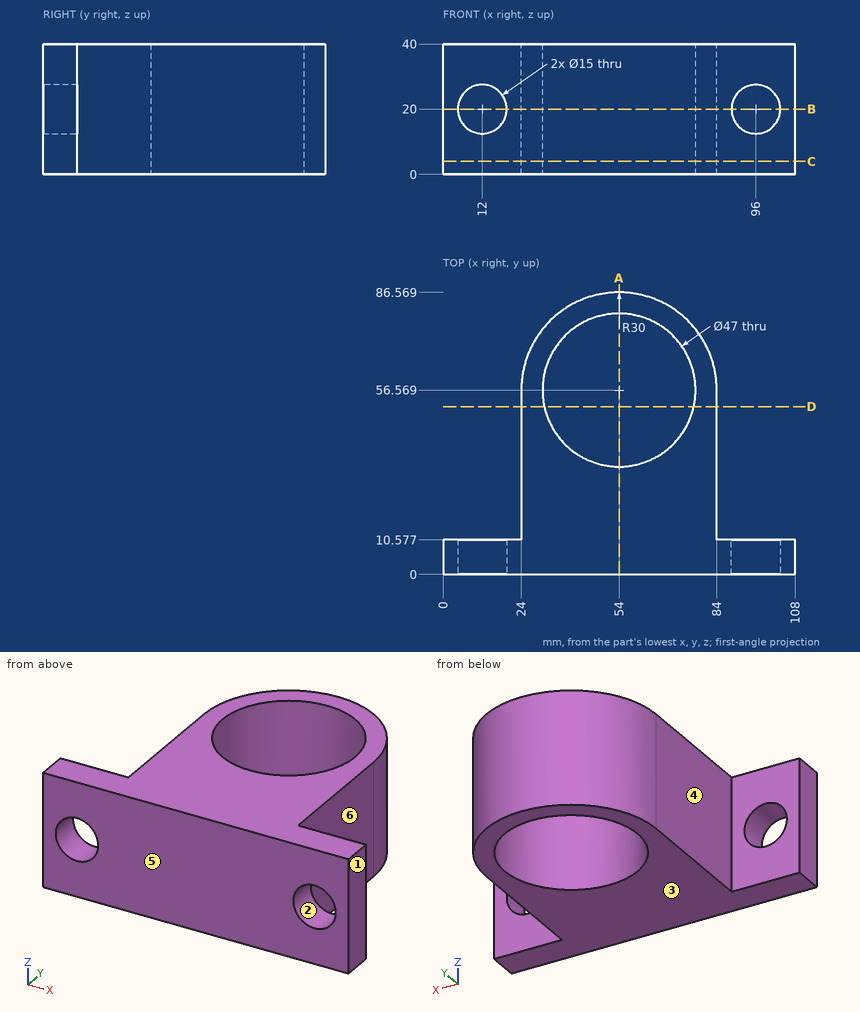
Job drawing, mm, ordinate dimensions from the low corner. One solid piece. A direction names the side the tool comes from. Coordinates: 2 decimals unless noted, no trailing zeros. Write each loop counter-clockwise with the first axis right and the second up, starting at its lowest first coordinate (ties: lowest second). Pieces come first, ordered by that corner, then holes. Notation, with made-up numbers: (-30.5, -12) - (7.5, -12) arc R33 cw to (7.5, 19) - close; hole circle Ø1 at (63.25, 89). An arc over 180 degrees is marked (long way). Use a Markdown table: item, result. Add a question column.
Item 1: Band-saw the part on B-B, the plane z = 20. Give the cut face in (x, y), and give its area (3 significant figures).
Item 2: 3-axis set-ups, long thin cutter, end or side, ignore diameter. For the marked faces 4, 5 and 6: which of +Z, -Z, +X, -X, +Y, -Y reach the whole face in a straight line?
Item 3: Band-saw the part on C-C, the plane z = 4. Give the cut face in (x, y).
Item 4: Flat gauge pins, fed straight in: pin 1 (1.5 mm diameter, centred on y = 66.5, z = 7, fed in from +X); pin 2 (10 mm diameter, centred on x = 39.5, y = 75, fed in from -Z); pin 3 (19 mm diameter, centred on x = 17.5, z = 26.5, fed in from +Y) (1 decimal); pin 4 (8 mm diameter, centred on y = 23.5, z = 7.5, fed in from -X). Where does each tip first touch, or does it go through?
Item 5: Band-saw the part on A-A, the plane x = 54. Give the cut face in (y, z).
Item 6: Mould opens along Z. For the marked faces 1, 2 and 3 say: pulls with the +Z half, pulls with the -Z half, needs draft (parallel to the pull), parting line crosses it, or undercut.
Item 7: Band-saw the part on D-D, the plane y = 51.5. Give the cut face in (x, z).
Item 8: Drill centre lines: L1, parallel to X at y = 8.75, z = 20; L2, parallel to Z at x = 96, y = 3; L3, parallel to X at y = 23, z = 7. Where is each one in solid material? Low to high. Write a range as from..to.
Numbers:
| question | item | result |
|---|---|---|
| 1 | outline | (0, 0) - (4.5, 0) - (4.5, 10.58) - (0, 10.58) - close; (19.5, 0) - (88.5, 0) - (88.5, 10.58) - (84, 10.58) - (84, 56.57) arc R30 ccw to (24, 56.57) - (24, 10.58) - (19.5, 10.58) - close; (103.5, 0) - (108, 0) - (108, 10.58) - (103.5, 10.58) - close; hole circle Ø47 at (54, 56.57) |
| 1 | area | 3,260 mm2 |
| 2 | face 4 | +Z, -Z, -X, +Y |
| 2 | face 5 | +Z, -Z, +X, -X, -Y |
| 2 | face 6 | +Z, -Z, +X, +Y |
| 3 | outline | (0, 0) - (108, 0) - (108, 10.58) - (84, 10.58) - (84, 56.57) arc R30 ccw to (24, 56.57) - (24, 10.58) - (0, 10.58) - close; hole circle Ø47 at (54, 56.57) |
| 4 | pin 1 | x = 82.56 |
| 4 | pin 2 | z = 0 |
| 4 | pin 3 | y = 69.6 |
| 4 | pin 4 | x = 24 |
| 5 | outline | (0, 0) - (33.07, 0) - (33.07, 40) - (0, 40) - close; (80.07, 0) - (86.57, 0) - (86.57, 40) - (80.07, 40) - close |
| 6 | face 1 | needs draft |
| 6 | face 2 | undercut |
| 6 | face 3 | pulls with the -Z half |
| 7 | outline | (24, 0) - (31.05, 0) - (31.05, 40) - (24, 40) - close; (76.95, 0) - (84, 0) - (84, 40) - (76.95, 40) - close |
| 8 | L1 | 0..4.5, 19.5..88.5, 103.5..108 |
| 8 | L2 | 0..12.5, 27.5..40 |
| 8 | L3 | 24..84 |
